```python
from build123d import *

# Parameters (mm, degrees)
EXTRUDE_1_DEPTH     = 25
EXTRUDE_2_DEPTH     = 104
CUT_EXTRUDE_1_DEPTH = 197.163197364
SKETCH_4_W          = 48
SKETCH_4_H          = 6.5
CUT_EXTRUDE_2_DEPTH = 3
SKETCH_5_R          = 8
CUT_EXTRUDE_3_DEPTH = 191.013157439
EXTRUDE_3_DEPTH     = 38


with BuildPart() as part:
    # Эскиз1 → Бобышка-Вытянуть1 (new body)
    with BuildSketch(Plane.XY):
        with BuildLine():
            Line((0, 0), (0, 136))
            Line((0, 136), (128, 136))
            Line((128, 136), (128, 0))
            Line((128, 0), (77.396182811, -64.769932368))
            ThreePointArc((77.396182811, -64.769932368), (64, -71.303687287), (50.603817189, -64.769932368))
            Line((50.603817189, -64.769932368), (0, 0))
        make_face()
    extrude(amount=EXTRUDE_1_DEPTH)

    # Эскиз2 → Бобышка-Вытянуть2 (add)
    with BuildSketch(Plane(origin=(0, 136, 0), x_dir=(1, 0, 0), z_dir=(0, 1, 0))):
        with BuildLine():
            Line((0, -25), (128, -25))
            ThreePointArc((128, -25), (64, -60), (0, -25))
        make_face()
    extrude(amount=-EXTRUDE_2_DEPTH)

    # Эскиз3 → Вырез-Вытянуть1 (cut, through all)
    with BuildSketch(Plane(origin=(128, 0, 0), x_dir=(0, 0, -1), z_dir=(1, 0, 0))):
        Polygon((-25, 32), (-60, 32), (-60, 82), align=None)
    extrude(amount=-CUT_EXTRUDE_1_DEPTH, mode=Mode.SUBTRACT)

    # Эскиз4 → Вырез-Вытянуть2 (cut)
    with BuildSketch(Plane(origin=(0, -1.22147651, 1.744966443), x_dir=(1, 0, 0), z_dir=(0, -0.5734623443633285, 0.8192319205190403))):
        with Locations((64, 76.801980066)):
            Rectangle(SKETCH_4_W, SKETCH_4_H)
    extrude(amount=-CUT_EXTRUDE_2_DEPTH, mode=Mode.SUBTRACT)

    # Эскиз5 → Вырез-Вытянуть3 (cut, through all)
    with BuildSketch(Plane.XY.offset(25)):
        with Locations((64, -54.303687287)):
            Circle(SKETCH_5_R)
    extrude(amount=-CUT_EXTRUDE_3_DEPTH, mode=Mode.SUBTRACT)

    # Эскиз6 → Бобышка-Вытянуть3 (add)
    with BuildSketch(Plane(origin=(0, 0, 0), x_dir=(-1, 0, 0), z_dir=(0, 0, -1))):
        Polygon((-128, 136), (0, 136), (0, 0), (-14.844426904, -19), (-113.155573096, -19), (-128, 0), align=None)
    extrude(amount=EXTRUDE_3_DEPTH)


solid = part.part
```
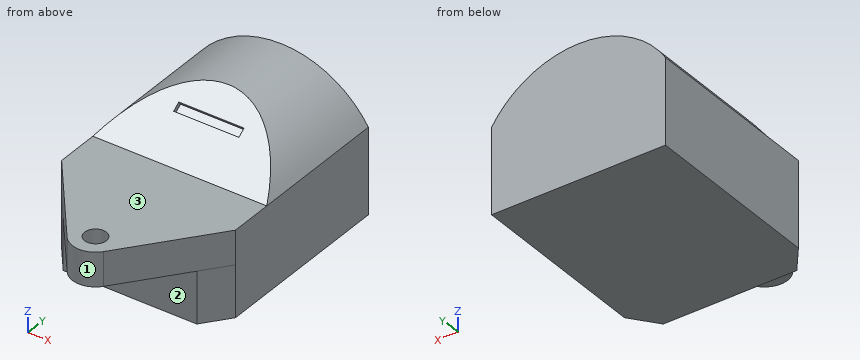
Work out the finished part from the listing and answer in its coordinate system (mm). Face numbers are marked on the shaded views. A direction names the side the tool comes from. Round coordinates to 2 decimals unless told otherwise and drop trailing zeros. Write each loop counter-clockwise with the first axis right and the second up, starting at its lowest first coordinate (ties: lowest second). Pieces come first, ordered by that corner, then holes.
1) A cutting plane is placed at D-D on y = -16. Determine the outline of the cut face in (x, z).
2) A cutting plane is placed at C-C on x = 17. Determine the outline of the cut face in (y, z), and give its area (3 significant figures).
3) Consider probe 1 along Y at (x, z) = (64, 17); probe 2 along Z at (x, y) = (106.5, -19.5); probe 3 along Z at (x, y) = (69.5, 15). Determine where each line is inside the solid, lowest interval first.
4) A cutting plane is placed at B-B on z = 8. Determine the outline of the cut face in (x, y).
5) Which of the six approach directions +Z, -Z, +X, -X, +Y, -Y give full straight-line access (tool end or side, diameter ignored) to the marked faces 1, 2 and 3?
6) A cutting plane is placed at A-A on x = 64. Determine the outline of the cut face in (y, z), and give its area (3 significant figures).
7) Flat-ended cylindrical pins translate along their axes: P1, Ø12, axis at x = 22.5, y = 16, coming from the +Z side; P2, Ø3, axis at y = 62, z = 44.5, coming from the +X side; P3, Ø5, axis at y = -25, z = 2, coming from the +X side. Find the tip coordinate at first contact, or state that the pin passes through.
Entries:
1. outline: (12.5, -38) - (115.5, -38) - (115.5, 25) - (12.5, 25) - close
2. outline: (-21.76, 0) - (-19, 0) - (-19, -38) - (136, -38) - (136, 43.73) - (58.75, 43.73) - (32, 25) - (-21.76, 25) - close
2. area: 11,500 mm2
3. probe 1: y = -71.3 to -62.3, -46.3 to 136
3. probe 2: z = 0 to 25
3. probe 3: z = -38 to 25
4. outline: (0, 0) - (50.6, -64.77) arc R17 ccw to (77.4, -64.77) - (128, 0) - (128, 136) - (0, 136) - close; hole circle Ø16 at (64, -54.3)
5. face 1: +Z, -Z, -Y
5. face 2: -Z, +X, -X, -Y
5. face 3: +Z, +X, -X, -Y
6. outline: (-71.3, 0) - (-62.3, 0) - (-62.3, 25) - (-71.3, 25) - close; (-46.3, 0) - (-19, 0) - (-19, -38) - (136, -38) - (136, 60) - (82, 60) - (64.36, 47.65) - (66.08, 45.19) - (60.76, 41.47) - (59.03, 43.92) - (32, 25) - (-46.3, 25) - close
6. area: 13,400 mm2
7. P1: stops at z = 25
7. P2: stops at x = 111.91
7. P3: stops at x = 110.42
